Geometry check sheet. Reference: the model listing, model coordinates, mm. Face numbers are marked on the shaded views. A direction names the side the tool comes from. Coordinates: 2 decimals unless noted, no trailing zeros. Loops run counter-clockwise (first coordinate to the right, second up) from the corner with the lowest first, then second, coordinate; pieces in that order, holes last. Notation, with made-up numbers: (17, 64) -> (61, 64) arc R25 cw to (61, 76) -> close; hole circle Ø10 at (-35.75, -31). An arc over 180 degrees is marked (long way). Answer as a JSON object with one key per item and string values.
from build123d import *

# Parameters (mm, degrees)
F0_W     = 425
F0_H     = 445
F0_W_2   = 345
F0_H_2   = 365
F1_DEPTH = 30
F2_R     = 8.25
F3_DEPTH = 80
F4_R     = 8.25
F5_DEPTH = 80
F6_W     = 60
F6_H     = 15
F7_DEPTH = 80


with BuildPart() as f1:
    # F0 (on Top) → F1 (new body, symmetric)
    with BuildSketch(Plane.XY):
        Rectangle(F0_W, F0_H)
        Rectangle(F0_W_2, F0_H_2, mode=Mode.SUBTRACT)
    extrude(amount=F1_DEPTH, both=True)

    # F2 (on face) → F3 (cut)
    with BuildSketch(Plane.XZ.offset(222.5)):
        with Locations((-60, 0)):
            Circle(F2_R)
        with Locations((60, 0)):
            Circle(F2_R)
    extrude(amount=-F3_DEPTH, mode=Mode.SUBTRACT)

    # F4 (on face) → F5 (cut)
    with BuildSketch(Plane.YZ.offset(212.5)):
        with Locations((60, 0)):
            Circle(F4_R)
        with Locations((-60, 0)):
            Circle(F4_R)
    extrude(amount=-F5_DEPTH, mode=Mode.SUBTRACT)

    # F6 (on face) → F7 (cut)
    with BuildSketch(Plane(origin=(0, 222.5, 0), x_dir=(-1, 0, 0), z_dir=(0, 1, 0))):
        Rectangle(F6_W, F6_H)
    extrude(amount=-F7_DEPTH, mode=Mode.SUBTRACT)


solid = f1.part
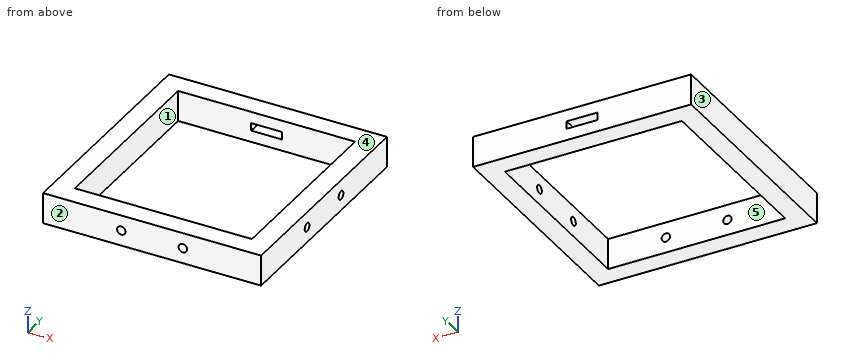
1. Section check A-A, the plane x = -60. Record the boundary of the cut face in (y, z), then the cut area to 3 significant figures.
Evaluation:
{"outline": "(-222.5, -30) -> (-182.5, -30) -> (-182.5, -8.25) -> (-222.5, -8.25) -> close; (-222.5, 8.25) -> (-182.5, 8.25) -> (-182.5, 30) -> (-222.5, 30) -> close; (182.5, -30) -> (222.5, -30) -> (222.5, 30) -> (182.5, 30) -> close", "area": "4,140 mm^2"}
2. Mould release check, pull along Y, two halves, no side actions. Record for the marked faces 1, 2 and 3: released by +Y, released by -Y, zero draft, split by the parting line, or undercut.
Evaluation:
{"face 1": "undercut", "face 2": "released by -Y", "face 3": "zero draft"}
3. Section check C-C, the plane y = -60. Record the boundary of the cut face in (x, z), then the cut area to 3 significant figures.
Evaluation:
{"outline": "(-212.5, -30) -> (-172.5, -30) -> (-172.5, 30) -> (-212.5, 30) -> close; (172.5, -30) -> (212.5, -30) -> (212.5, -8.25) -> (172.5, -8.25) -> close; (172.5, 8.25) -> (212.5, 8.25) -> (212.5, 30) -> (172.5, 30) -> close", "area": "4,140 mm^2"}
4. Tool access check on the marked faces 4 and 5. Record the directions out of +Z, -Z, +X, -X, +Y, -Y that give a thin tool (end or side, any length) a straight path to the whole face; none if there is none.
Evaluation:
{"face 4": "+Z, +X, -X, +Y, -Y", "face 5": "+Z, -Z"}
5. Depth check by flat-ended pin: P1, Ø13, axis at y = -60, z = 0, coming from the +X side. Enter the tip coordinate at first touch or a pass-through.
Evaluation:
{"P1": "stops at x = -172.5"}
6. Section check B-B, the plane z = 0. Record the boundary of the cut face in (x, y), then the cut area to 3 significant figures.
Evaluation:
{"outline": "(-212.5, -222.5) -> (-68.25, -222.5) -> (-68.25, -182.5) -> (-172.5, -182.5) -> (-172.5, 182.5) -> (-30, 182.5) -> (-30, 222.5) -> (-212.5, 222.5) -> close; (-51.75, -222.5) -> (51.75, -222.5) -> (51.75, -182.5) -> (-51.75, -182.5) -> close; (30, 182.5) -> (172.5, 182.5) -> (172.5, 68.25) -> (212.5, 68.25) -> (212.5, 222.5) -> (30, 222.5) -> close; (68.25, -222.5) -> (212.5, -222.5) -> (212.5, -68.25) -> (172.5, -68.25) -> (172.5, -182.5) -> (68.25, -182.5) -> close; (172.5, -51.75) -> (212.5, -51.75) -> (212.5, 51.75) -> (172.5, 51.75) -> close", "area": "58,200 mm^2"}
7. Thickness scan on probe 1 along X at (y, z) = (-22.5, -10.5); probe 2 along Y at (x, z) = (-162, -14); probe 3 along Z at (x, y) = (187, -60). Record the ranges inside material, lowest first. Write a range as from..to.
Evaluation:
{"probe 1": "x = -212.5..-172.5, 172.5..212.5", "probe 2": "y = -222.5..-182.5, 182.5..222.5", "probe 3": "z = -30..-8.25, 8.25..30"}
8. Section check D-D, the plane x = -144. Record the boundary of the cut face in (y, z), then the cut area to 3 significant figures.
Evaluation:
{"outline": "(-222.5, -30) -> (-182.5, -30) -> (-182.5, 30) -> (-222.5, 30) -> close; (182.5, -30) -> (222.5, -30) -> (222.5, 30) -> (182.5, 30) -> close", "area": "4,800 mm^2"}
